Geometry: final body of the model. Coordinates: model frame, mm. A direction names the side the tool comes from. Round coordinates to 2 decimals unless told otherwise and drop trailing zeros. Loops run counter-clockwise (first coordinate to the right, second up) from the corner with the lowest first, then second, coordinate; pieces in that order, holes last. Notation, with made-up numbers: (1.25, 21.5) -> (7.25, 21.5) arc R25 ccw to (7.25, 57.5) -> close; hole circle Ø6 at (-8, 37.25). An arc over 180 degrees is marked (long way). Answer in a Markdown table with one row per item.
```python
from build123d import *

# Parameters (mm, degrees)
F0_R     = 9.5
F1_DEPTH = 3


with BuildPart() as f1:
    # F0 (on Top) → F1 (new body)
    with BuildSketch(Plane.XY):
        Polygon((11.243366, 11.103062), (9.021332, 15.101957), (8.113263, 15.101957), (13.079281, 23.516777), (6.958124, 35.085378), (-6.121157, 35.568601), (-13.079281, 24.483223), (-7.813124, 15.101957), (-8.187056, 15.101957), (-11.144701, 11.158155), (-15.099014, 8.810067), (-15.099014, 7.820336), (-24.48028, 13.086494), (-35.565659, 6.12837), (-35.082436, -6.950911), (-23.513834, -13.072069), (-15.099014, -8.10605), (-15.099014, -9.01412), (-11.071869, -11.280808), (-8.187056, -15.101957), (-7.813124, -15.101957), (-13.079281, -24.483223), (-6.121157, -35.568601), (6.958124, -35.085378), (13.079281, -23.516777), (8.113263, -15.101957), (9.021332, -15.101957), (11.17502, -11.226061), (15.1049, -9.01412), (15.1049, -8.10605), (23.51972, -13.072069), (35.088321, -6.950911), (35.571544, 6.12837), (24.486166, 13.086494), (15.1049, 7.820336), (15.1049, 8.810067), align=None)
        with Locations((0, -24)):
            Circle(F0_R, mode=Mode.SUBTRACT)
        with Locations((-23.997057, 0.007213)):
            Circle(F0_R, mode=Mode.SUBTRACT)
        with BuildLine():
            ThreePointArc((-11, 0), (0, 11), (11, 0))
            ThreePointArc((11, 0), (0, -11), (-11, 0))
        make_face(mode=Mode.SUBTRACT)
        with Locations((0, 24)):
            Circle(F0_R, mode=Mode.SUBTRACT)
        with Locations((24.002943, 0.007213)):
            Circle(F0_R, mode=Mode.SUBTRACT)
    extrude(amount=F1_DEPTH)


solid = f1.part
```
Item 1: Line query: probe 1 along Y at (x, z) = (0, 1); probe 2 along X at (y, z) = (-5.5, 1.85); probe 3 along X at (y, z) = (-4, 0.3). Output: solid intervals per line, ascending. Write a range as [from, to].
Answer:
| item | result |
|---|---|
| probe 1 | y = [-35.34, -33.5], [-14.5, -11], [11, 14.5], [33.5, 35.34] |
| probe 2 | x = [-35.14, -31.74], [-16.26, -9.53], [9.53, 16.26], [31.74, 35.14] |
| probe 3 | x = [-35.19, -32.61], [-15.38, -10.25], [10.25, 15.39], [32.62, 35.2] |
Item 2: Cut plane B-B (x = 0). Output: boundary loops of the cut face in (y, z).
Answer:
| item | result |
|---|---|
| outline | (-35.34, 0) -> (-33.5, 0) -> (-33.5, 3) -> (-35.34, 3) -> close; (-14.5, 0) -> (-11, 0) -> (-11, 3) -> (-14.5, 3) -> close; (11, 0) -> (14.5, 0) -> (14.5, 3) -> (11, 3) -> close; (33.5, 0) -> (35.34, 0) -> (35.34, 3) -> (33.5, 3) -> close |
Item 3: Cut plane D-D (y = -1.5). Output: boundary loops of the cut face in (x, z), then the cut area to 3 significant figures.
Answer:
| item | result |
|---|---|
| outline | (-35.28, 0) -> (-33.38, 0) -> (-33.38, 3) -> (-35.28, 3) -> close; (-14.62, 0) -> (-10.9, 0) -> (-10.9, 3) -> (-14.62, 3) -> close; (10.9, 0) -> (14.62, 0) -> (14.62, 3) -> (10.9, 3) -> close; (33.38, 0) -> (35.29, 0) -> (35.29, 3) -> (33.38, 3) -> close |
| area | 33.8 mm² |
Item 4: Reachability of faces 1 (the face through (-29.38, -9.97, 1.48)), 2 (the face through (-10.41, -19.73, 1.48)), 3 (the face through (-13.114, -10.132, 1.479)), 4 (the face through (10.56, 19.25, 1.48)), 5 (the face through (-19.365, -10.624, 1.479)) from +Z, -Z, +X, -X, +Y, -Y: full face, straight path, thin tool, end or side. Return the list, or none.
Answer:
| item | result |
|---|---|
| face 1 | +Z, -Z, -X, -Y |
| face 2 | +Z, -Z, -X |
| face 3 | +Z, -Z |
| face 4 | +Z, -Z, +X |
| face 5 | +Z, -Z, -Y |
Item 5: Draft query along X for faces 6 (the face through (-3, 11, 3)), 7 (the face through (10.083, -13.191, 1.479)), 8 (the face through (10.63, -19.37, 1.48)). Return one class per face: pulls with the +X half, pulls with the -X half, needs draft (parallel to the pull), parting line crosses it, or undercut.
Answer:
| item | result |
|---|---|
| face 6 | needs draft |
| face 7 | undercut |
| face 8 | pulls with the +X half |
Item 6: Cut plane C-C (x = -16). Output: boundary loops of the cut face in (y, z), then the cut area to 3 significant figures.
Answer:
| item | result |
|---|---|
| outline | (-8.64, 0) -> (-5.12, 0) -> (-5.12, 3) -> (-8.64, 3) -> close; (5.14, 0) -> (8.33, 0) -> (8.33, 3) -> (5.14, 3) -> close |
| area | 20.1 mm² |
Item 7: Cut plane A-A (y = 16). Output: boundary loops of the cut face in (x, z), then the cut area to 3 significant figures.
Answer:
| item | result |
|---|---|
| outline | (-8.32, 0) -> (-5.12, 0) -> (-5.12, 3) -> (-8.32, 3) -> close; (5.12, 0) -> (8.64, 0) -> (8.64, 3) -> (5.12, 3) -> close |
| area | 20.1 mm² |
Item 8: Pin query (flat end, axial travel): pin 1 Ø0.5 at (x, z) = (9, 2) entering from -Y; pin 2 Ø1 at (y, z) = (-8.5, 2) entering from -X; pin 3 Ø1 at (y, z) = (-8.5, 1) entering from +X. Return the tip coordinate at first contact, or that it passes through.
Answer:
| item | result |
|---|---|
| pin 1 | stops at y = -31.7 |
| pin 2 | stops at x = -33.1 |
| pin 3 | stops at x = 33.11 |
